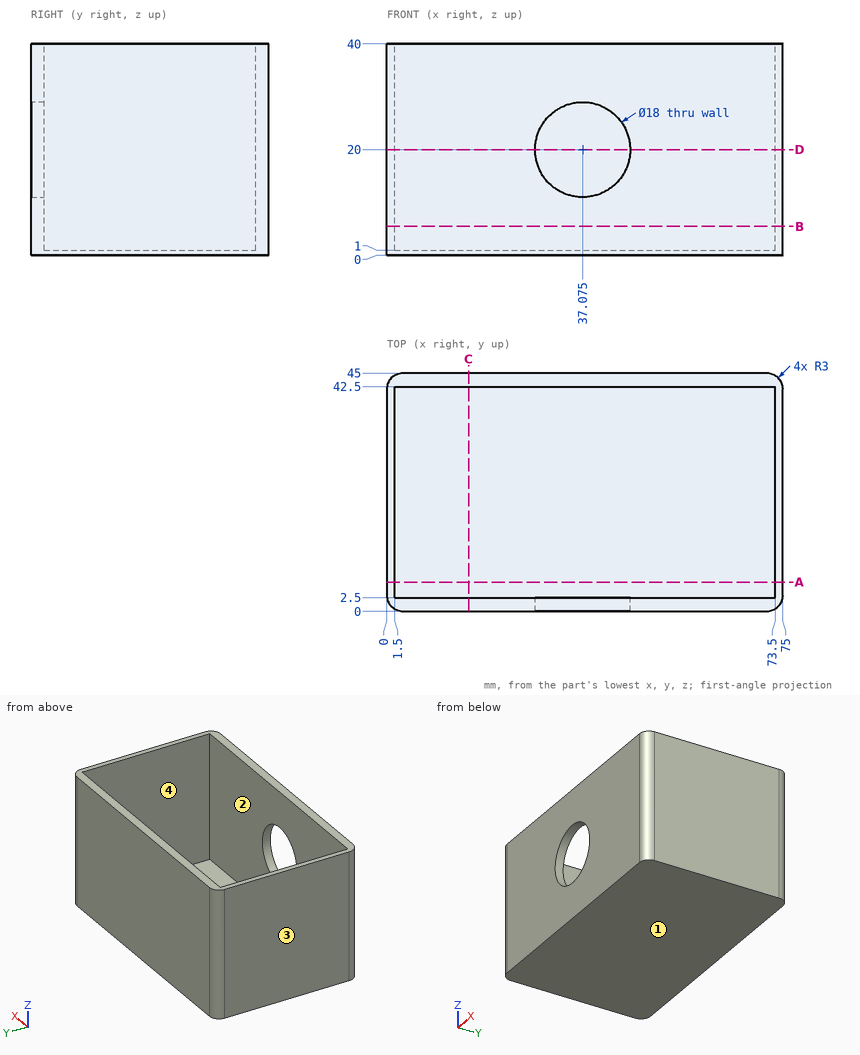
The drawing under review shows one solid part. Ordinate dimensions are in mm from its lowest x, y, z. Coordinates: 2 decimals unless noted, no trailing zeros. Write each loop counter-clockwise with the first axis right and the second up, starting at its lowest first coordinate (ties: lowest second). Pieces come first, ordered by that corner, then holes.
1) Add section C-C (x = 15.5). Write out the cut boundary in (y, z).
2) To check wall thickness, follow L1, parallel to X at y = 27.5, z = 5; L2, parallel to Y at x = 60.5, z = 19.5; L3, parallel to Z at x = 43, y = 41. State the ranges of each line that lie inside material, in increasing order.
3) Add section A-A (y = 5.5). Write out the cut boundary in (x, z), plus the area to 3 significant figures.
4) Add section D-D (z = 20). Write out the cut boundary in (x, y) (3 decimals).
5) Add section B-B (z = 5.5). Write out the cut boundary in (x, y).
6) Insertion check: pin 1 (10 mm diameter, centred on x = 31, y = 19, fed in from +Z). The pin has a flat end and moves straight along its axis. Give the tip position at first contact, or say it passes through.
7) Mouldability with a two-part tool opening along X and no side actions: class the marked faces 1, 2, 3 and 4 as +X half, -X half, draft (parallel to the pull), parting line (faces both ways), or undercut.
Check result:
1. outline: (0, 0) - (45, 0) - (45, 40) - (42.5, 40) - (42.5, 1) - (2.5, 1) - (2.5, 40) - (0, 40) - close
2. L1: x = 0 to 1.5, 73.5 to 75
2. L2: y = 0 to 2.5, 42.5 to 45
2. L3: z = 0 to 1
3. outline: (0, 0) - (75, 0) - (75, 40) - (73.5, 40) - (73.5, 1) - (1.5, 1) - (1.5, 40) - (0, 40) - close
3. area: 192 mm2
4. outline: (0, 3) arc R3 ccw to (3, 0) - (28.075, 0) - (28.075, 2.5) - (1.5, 2.5) - (1.5, 42.5) - (73.5, 42.5) - (73.5, 2.5) - (46.075, 2.5) - (46.075, 0) - (72, 0) arc R3 ccw to (75, 3) - (75, 42) arc R3 ccw to (72, 45) - (3, 45) arc R3 ccw to (0, 42) - close
5. outline: (0, 3) arc R3 ccw to (3, 0) - (72, 0) arc R3 ccw to (75, 3) - (75, 42) arc R3 ccw to (72, 45) - (3, 45) arc R3 ccw to (0, 42) - close; hole (1.5, 2.5) - (73.5, 2.5) - (73.5, 42.5) - (1.5, 42.5) - close
6. pin 1: stops at z = 1
7. face 1: draft
7. face 2: undercut
7. face 3: -X half
7. face 4: undercut
